Read the model definition and answer for the solid it produces. Units are mm, in the model's axes. Face numbers are marked on the shaded views. A direction names the side the tool comes from. Give positions to 0.01 mm unless a question says otherwise; leave off trailing zeros. Write each loop counter-clockwise with the first axis right and the second up, starting at its lowest first coordinate (ties: lowest second). Pieces come first, ordered by that corner, then holes. Notation, with made-up numbers: (61, -13) -> (95, -13) arc R11 ccw to (95, -8) -> close; hole circle Ø4 at (65.25, 8). An arc over 180 degrees is marked (long way). Write item = value, one per line.
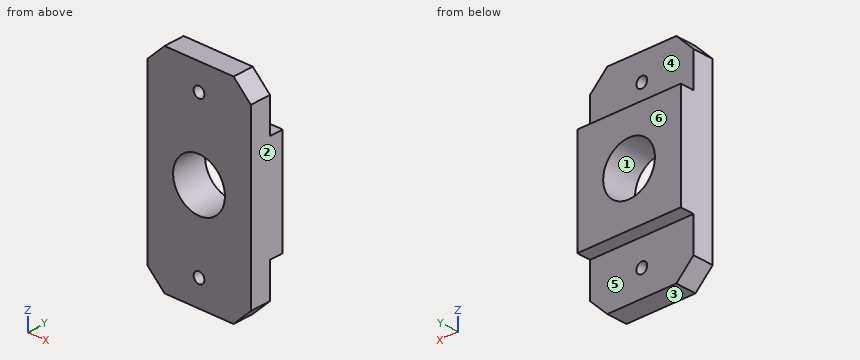
from build123d import *

# Parameters (mm, degrees)
SKETCH1_W           = 76.2
SKETCH1_H           = 76.2
BOSS_EXTRUDE1_DEPTH = 7.62
SKETCH2_W           = 38.1
SKETCH2_H           = 38.1
BOSS_EXTRUDE2_DEPTH = 5.08
SKETCH3_R           = 9.525
CUT_EXTRUDE1_DEPTH  = 13.7
SKETCH4_R           = 1.984375
CUT_EXTRUDE2_DEPTH  = 13.7
CUT_EXTRUDE3_DEPTH  = 8.62
CHAMFER1_SIZE       = 6.35


with BuildPart() as part:
    # Sketch1 → Boss-Extrude1 (new body)
    with BuildSketch(Plane(origin=(0, 0, 0), x_dir=(1, 0, 0), z_dir=(0, 1, 0))):
        Rectangle(SKETCH1_W, SKETCH1_H)
    extrude(amount=BOSS_EXTRUDE1_DEPTH)

    # Sketch2 → Boss-Extrude2 (add)
    with BuildSketch(Plane(origin=(0, 7.62, 0), x_dir=(1, 0, 0), z_dir=(0, 1, 0))):
        Rectangle(SKETCH2_W, SKETCH2_H)
    extrude(amount=BOSS_EXTRUDE2_DEPTH)

    # Sketch3 → Cut-Extrude1 (cut, through all)
    with BuildSketch(Plane(origin=(0, 12.7, 0), x_dir=(1, 0, 0), z_dir=(0, 1, 0))):
        Circle(SKETCH3_R)
    extrude(amount=-CUT_EXTRUDE1_DEPTH, mode=Mode.SUBTRACT)

    # Sketch4 → Cut-Extrude2 (cut, through all)
    with BuildSketch(Plane(origin=(0, 12.7, 0), x_dir=(1, 0, 0), z_dir=(0, 1, 0))):
        with Locations((0, 28.575)):
            Circle(SKETCH4_R)
        with Locations((0, -28.575)):
            Circle(SKETCH4_R)
    extrude(amount=-CUT_EXTRUDE2_DEPTH, mode=Mode.SUBTRACT)

    # Sketch5 → Cut-Extrude3 (cut, through all)
    with BuildSketch(Plane(origin=(0, 7.62, 0), x_dir=(1, 0, 0), z_dir=(0, 1, 0))):
        Polygon((-38.1, -38.1), (-19.05, -38.1), (-19.05, 19.05), (-19.05, 38.1), (-38.1, 38.1), (-38.1, 19.05), align=None)
        Polygon((19.05, 38.1), (19.05, 19.05), (19.05, -38.1), (38.1, -38.1), (38.1, 19.05), (38.1, 38.1), align=None)
    extrude(amount=-CUT_EXTRUDE3_DEPTH, mode=Mode.SUBTRACT)

    # Chamfer1
    chamfer1_edges = [part.edges().sort_by_distance(p)[0] for p in [
        (-19.05, 3.81, -38.1),
        (-19.05, 3.81, 38.1),
        (19.05, 3.81, -38.1),
        (19.05, 3.81, 38.1),
    ]]
    chamfer(chamfer1_edges, length=CHAMFER1_SIZE)


solid = part.part
(1) The part is cut by section C-C on x = -6. Determine the outline of the cut face in (y, z).
Checks:
outline = (0, -38.1) -> (7.62, -38.1) -> (7.62, -19.05) -> (12.7, -19.05) -> (12.7, -7.4) -> (0, -7.4) -> close; (0, 7.4) -> (12.7, 7.4) -> (12.7, 19.05) -> (7.62, 19.05) -> (7.62, 38.1) -> (0, 38.1) -> close
(2) Consider L1, parallel to Z at x = 0, y = 2 (3 decimals); L2, parallel to X at y = 5, z = 0 (3 decimals); L3, parallel to Y at x = 7, z = -21. Determine where each line is inside the solid, lowest interval first.
Checks:
L1 = -38.1 to -30.559, -26.591 to -9.525, 9.525 to 26.591, 30.559 to 38.1
L2 = -19.05 to -9.525, 9.525 to 19.05
L3 = 0 to 7.62
(3) The part is cut by section D-D on y = 3.5. Determine the outline of the cut face in (x, z) (3 decimals).
Checks:
outline = (-19.05, -31.75) -> (-12.7, -38.1) -> (12.7, -38.1) -> (19.05, -31.75) -> (19.05, 31.75) -> (12.7, 38.1) -> (-12.7, 38.1) -> (-19.05, 31.75) -> close; hole circle Ø19.05 at (0, 0); hole circle Ø3.969 at (0, -28.575); hole circle Ø3.969 at (0, 28.575)
(4) A tool of negligible diameter and unlimited length cuts with its end or side. For the marked faces 4, 5 and 6, from which of +Z, -Z, +X, -X, +Y, -Y can it reach the whole face along a straight path? Write none if from no direction.
Checks:
face_4 = +Z, +X, -X, +Y
face_5 = -Z, +X, -X, +Y
face_6 = +Z, -Z, +X, -X, +Y
(5) Given P1, Ø1.5, axis at x = -1.5, y = 9.5, coming from the +Z side; P2, Ø9.5, axis at x = -2, z = -33, coming from the +Y side; P3, Ø5.5, axis at x = 9, y = 9.5, coming from the -Z side, each flat-ended and moving along its own axis, determine where each tip first touches the part or whether it passes through.
Checks:
P1 = 19.05
P2 = 7.62
P3 = -38.1
(6) The part is cut by section A-A on x = 0. Determine the outline of the cut face in (y, z) (3 decimals), plus the area to 3 significant figures.
Checks:
outline = (0, -38.1) -> (7.62, -38.1) -> (7.62, -30.559) -> (0, -30.559) -> close; (0, -26.591) -> (7.62, -26.591) -> (7.62, -19.05) -> (12.7, -19.05) -> (12.7, -9.525) -> (0, -9.525) -> close; (0, 9.525) -> (12.7, 9.525) -> (12.7, 19.05) -> (7.62, 19.05) -> (7.62, 26.591) -> (0, 26.591) -> close; (0, 30.559) -> (7.62, 30.559) -> (7.62, 38.1) -> (0, 38.1) -> close
area = 472 mm²
(7) For a pull along X with two mould halves and no side action, classify the marked faces 1, 2 and 3 as released by +X, released by -X, zero draft, split by the parting line, or undercut.
Checks:
face_1 = undercut
face_2 = released by +X
face_3 = zero draft
(8) The part is cut by section B-B on z = 0. Determine the outline of the cut face in (x, y) (3 decimals), plus the area to 3 significant figures.
Checks:
outline = (-19.05, 0) -> (-9.525, 0) -> (-9.525, 12.7) -> (-19.05, 12.7) -> close; (9.525, 0) -> (19.05, 0) -> (19.05, 12.7) -> (9.525, 12.7) -> close
area = 242 mm²
